from build123d import *

# Parameters (mm, degrees)
F0_W     = 250
F0_H     = 100
F1_DEPTH = 20
F2_W     = 50
F2_H     = 75
F2_W_2   = 44
F2_H_2   = 69
F3_DEPTH = 800
F4_W     = 50
F4_H     = 75
F4_W_2   = 44
F4_H_2   = 69
F5_DEPTH = 837.2
F6_F1_R  = 1.5
F6_F2_R  = 1.5
F6_F3_R  = 1.5
F6_F4_R  = 1.4999


# Not quite as in the source:
# - a fillet or chamfer is up to 0.001 mm smaller than in the source, because OpenCascade refuses the exact size


with BuildPart() as f1:
    # F0 (on Top) → F1 (new body)
    with BuildSketch(Plane.XY):
        Rectangle(F0_W, F0_H)
    extrude(amount=F1_DEPTH)

    # F2 (on face) → F3 (join)
    with BuildSketch(Plane.XY.offset(20)):
        Rectangle(F2_W, F2_H)
        Rectangle(F2_W_2, F2_H_2, mode=Mode.SUBTRACT)
    extrude(amount=F3_DEPTH)

    # F4 (on face) → F5 (join)
    with BuildSketch(Plane.XZ.offset(37.5)):
        with Locations((0, 857.5)):
            Rectangle(F4_W, F4_H)
        with Locations((0, 857.5)):
            Rectangle(F4_W_2, F4_H_2, mode=Mode.SUBTRACT)
    extrude(amount=-F5_DEPTH)

    # F6: fillet of radius 1.5 on 44 edges, made by hand

    # F6_f1
    f6_f1_edges = [f1.edges().sort_by_distance(p)[0] for p in [
        (-22, -34.5, 420),
        (22, 34.5, 420),
        (22, -34.5, 420),
        (-22, 34.5, 420),
        (-22, 381.1, 892),
        (22, 381.1, 892),
        (0, 37.5, 820),
        (22, 381.1, 823),
        (-22, 381.1, 823),
        (22, 0, 820),
        (0, -34.5, 820),
        (-22, 0, 820),
        (0, 34.5, 820),
        (0, 34.5, 20),
        (-22, 0, 20),
        (22, 0, 20),
        (0, -34.5, 20),
    ]]
    fillet(f6_f1_edges, radius=F6_F1_R)

    # F6_f2
    f6_f2_edges = [f1.edges().sort_by_distance(p)[0] for p in [
        (-25, -37.5, 457.5),
        (25, 37.5, 419.25),
        (25, -37.5, 457.5),
        (-25, 37.5, 419.25),
        (25, 381.1, 895),
        (-25, 381.1, 895),
        (0, -37.5, 895),
        (125, -50, 10),
        (-125, -50, 10),
        (125, 50, 10),
        (0, -50, 0),
        (0, -50, 20),
        (0, 50, 20),
        (125, 0, 20),
        (-125, 0, 20),
        (-125, 50, 10),
        (0, 50, 0),
        (125, 0, 0),
        (-125, 0, 0),
        (-25, 37.9393398282, 819.5606601718),
        (25, 37.9393398282, 819.5606601718),
    ]]
    fillet(f6_f2_edges, radius=F6_F2_R)

    # F6_f3
    f6_f3_edges = [f1.edges().sort_by_distance(p)[0] for p in [
        (25, 0, 20),
        (-25, 0, 20),
        (0, -37.5, 20),
        (0, 37.5, 20),
        (24.5606601718, 37.0606601718, 20),
        (-24.5606601718, 37.0606601718, 20),
        (-24.5606601718, -37.0606601718, 20),
        (24.5606601718, -37.0606601718, 20),
    ]]
    fillet(f6_f3_edges, radius=F6_F3_R)

    # F6_f4 (radius 1.5 in the source; OpenCascade refuses exactly that, so slightly less here)
    f6_f4_edges = [f1.edges().sort_by_distance(p)[0] for p in [
        (-22, -37.5, 857.5),
        (0, -37.5, 823),
        (0, -37.5, 892),
        (22, -37.5, 857.5),
        (21.5606601718, -37.5, 891.5606601718),
        (21.5606601718, -37.5, 823.4393398282),
        (-21.5606601718, -37.5, 891.5606601718),
        (-21.5606601718, -37.5, 823.4393398282),
    ]]
    fillet(f6_f4_edges, radius=F6_F4_R)


solid = f1.part
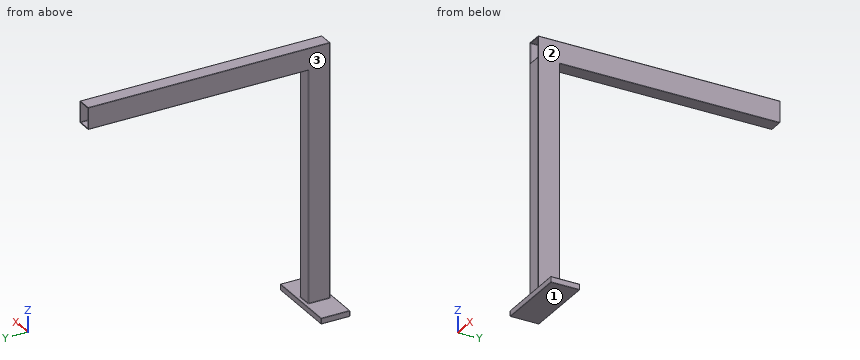
Read the model definition and answer for the solid it produces. Units are mm, in the model's axes. Face numbers are marked on the shaded views. A direction names the side the tool comes from. Give positions to 0.01 mm unless a question says otherwise; leave off trailing zeros. Write each loop counter-clockwise with the first axis right and the second up, starting at its lowest first coordinate (ties: lowest second). Pieces come first, ordered by that corner, then holes. Notation, with made-up numbers: M -28.5,87 L 10.5,87 A17 cw 10.5,97 Z; hole C 39,-24 d9. An arc over 180 degrees is marked long. One line per item, written item: value. Start each with the question number.
(1) Flat-ended cylindrical pins translate along their axes: pin 1 Ø12.5 at (x, y) = (-9, 368.5) entering from -Z; pin 2 Ø20.5 at (x, y) = (-7.5, 6.5) entering from -Z; pin 3 Ø18.5 at (x, z) = (10.5, 10.5) entering from +Y; pin 4 Ø20.5 at (x, z) = (3, 537) entering from +Y. Find the tip coordinate at first contact, or state that the pin passes through.
(2) Find section A-A (x = 7.5). Give the number of separate pieces and of enclosed holes in the cut face, plus the area to 3 significant figures.
(3) Find section C-C (z = 652). Determine the outline of the cut face in (x, y), plus the area to 3 significant figures.
(4) Find the intervals of material crossed by line 1 (Z direction, x = -19.5, y = 734); line 2 (X direction, y = -6.5, z = 393); line 3 (Y direction, x = 6, z = 265), in increasing order.
(5) A tool of negligible diameter and unlimited length cuts with its end or side. For the marked faces 1, 2 and 3, from which of +Z, -Z, +X, -X, +Y, -Y can it reach the whole face along a straight path? Write none if from no direction.
(6) Find section B-B (y = 348). Determine the outline of the cut face in (x, z).
(7) Find section D-D (x = -100). Determine the outline of the cut face in (y, z), plus the area to 3 significant figures.
Results below:
1. pin 1: stops at z = 820
1. pin 2: stops at z = 0
1. pin 3: stops at y = 50
1. pin 4: stops at y = 37.5
2. separate pieces: 2
2. enclosed holes: 1
2. area: 11,800 mm^2
3. outline: M -25,-36 A1.5 ccw -23.5,-37.5 L 23.5,-37.5 A1.5 ccw 25,-36 L 25,36 A1.5 ccw 23.5,37.5 L -23.5,37.5 A1.5 ccw -25,36 Z; hole M -22,-33 A1.5 ccw -20.5,-34.5 L 20.5,-34.5 A1.5 ccw 22,-33 L 22,33 A1.5 ccw 20.5,34.5 L -20.5,34.5 A1.5 ccw -22,33 Z
3. area: 714 mm^2
4. line 1: z = 820 to 823, 892 to 895
4. line 2: x = -25 to -22, 22 to 25
4. line 3: y = -37.5 to -34.5, 34.5 to 37.5
5. face 1: -Z, +X, -X, +Y, -Y
5. face 2: +Z, +X, +Y, -Y
5. face 3: +Z, -X, +Y, -Y
6. outline: M -25,821.5 A1.5 ccw -23.5,820 L 23.5,820 A1.5 ccw 25,821.5 L 25,893.5 A1.5 ccw 23.5,895 L -23.5,895 A1.5 ccw -25,893.5 Z; hole M -22,824.5 A1.5 ccw -20.5,823 L 20.5,823 A1.5 ccw 22,824.5 L 22,890.5 A1.5 ccw 20.5,892 L -20.5,892 A1.5 ccw -22,890.5 Z
7. outline: M -50,1.5 A1.5 ccw -48.5,0 L 48.5,0 A1.5 ccw 50,1.5 L 50,18.5 A1.5 ccw 48.5,20 L -48.5,20 A1.5 ccw -50,18.5 Z
7. area: 2,000 mm^2
